Read the model definition and answer for the solid it produces. Units are mm, in the model's axes. Face numbers are marked on the shaded views. Give positions to 0.01 mm unless a question says otherwise; leave off trailing zeros. Order: outer loops, then holes, each group sorted by start corner. A loop starts at its lowest first (then second) coordinate and runs counter-clockwise, first axis right, second up. Notation, with made-up numbers: (50.5, -38) - (95.5, -38) arc R12 ccw to (95.5, -28) - close; hole circle Ø8 at (67.25, 71). An arc over 180 degrees is marked (long way). Return JSON: item names as keys, results as strings.
```python
from build123d import *

# Parameters (mm, degrees)
SHELL3_T           = 10
SKETCH5_R          = 8.5
CUT_EXTRUDE1_DEPTH = 10
CHAMFER2_SIZE      = 5


with BuildPart() as part:
    # Sketch4 → Loft3 section 0
    with BuildSketch(Plane(origin=(120, 0, 0), x_dir=(0, 0, -1), z_dir=(1, 0, 0))):
        with BuildLine():
            Line((13.75, 7.5), (-13.75, 7.5))
            Line((-13.75, 7.5), (-13.75, 32.5))
            Line((-13.75, 32.5), (13.75, 32.5))
            Line((13.75, 32.5), (13.75, 7.5))
        make_face()
    # Sketch1 → Loft3 section 1
    with BuildSketch(Plane(origin=(0, 0, 0), x_dir=(0, 0, -1), z_dir=(1, 0, 0))):
        with BuildLine():
            Line((-13.625, -12.5), (13.625, -12.5))
            Line((13.625, -12.5), (13.625, 12.5))
            Line((13.625, 12.5), (-13.625, 12.5))
            Line((-13.625, 12.5), (-13.625, -12.5))
        make_face()
    loft()

    # Shell3
    shell3_openings = [part.faces().sort_by_distance(p)[0] for p in [
        (60.091324201, 22.5152207, 0),
        (120, 20, 0),
    ]]
    offset(amount=SHELL3_T, openings=shell3_openings, kind=Kind.INTERSECTION)

    # Sketch5 → Cut-Extrude1 (cut)
    with BuildSketch(Plane(origin=(2.027027027, -12.162162162, 0), x_dir=(0.9863939238321439, 0.1643989873053572, 0), z_dir=(-0.1643989873053572, 0.9863939238321439, 0))):
        with Locations(Location((8.494520618, 0, 0), (0, 0, 180))):
            Circle(SKETCH5_R)
    extrude(amount=-CUT_EXTRUDE1_DEPTH, mode=Mode.SUBTRACT)

    # Chamfer2
    # the kernel refuses this chamfer: 5 mm, written as the material it takes off along each edge
    with BuildSketch(Plane(origin=(10.40597055, -10.765671575, 0), x_dir=(-0.9863939238321437, -0.1643989873053573, 0), z_dir=(0, 0, -1))) as chamfer2_piece_1_section:
        Polygon((8.5 + CHAMFER2_SIZE, 0), (8.5, -CHAMFER2_SIZE), (8.5, 0), align=None)
    chamfer2_piece_1 = revolve(axis=Axis((10.40597055, -10.765671575, 0), (-0.1643989873053572, 0.9863939238321439, 0)), mode=Mode.PRIVATE)
    chamfer2_piece_1 = split(chamfer2_piece_1, bisect_by=Plane(origin=(0, -11.368477015, 0), z_dir=(1, 0, 0)), keep=Keep.TOP, mode=Mode.PRIVATE)
    add(chamfer2_piece_1, mode=Mode.SUBTRACT)


solid = part.part
```
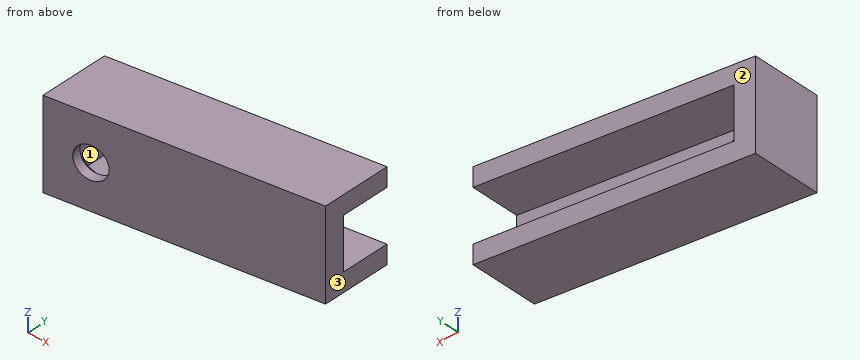
Q1. A cutting plane is placed at A-A (z = 20.5). Write down the section's boundary in (x, y).
Values:
{"outline": "(-10, -24.3) - (120, -2.64) - (120, 32.5) - (-10, 10.83) - close"}
Q2. Consider L1, parallel to Z at x = 108, y = 6; L2, parallel to Z at x = 105.5, y = 5; L3, parallel to Z at x = 21, y = 0. Determine where each line is inside the solid, lowest interval first.
Values:
{"L1": "z = -23.74 to -13.74, 13.74 to 23.74", "L2": "z = -23.73 to 23.73", "L3": "z = -23.65 to -13.65, 13.65 to 23.65"}
Q3. Given pin 1 (1.5 mm diameter, centred on x = 81, z = -1.5, fed in from -Y); pin 2 (8 mm diameter, centred on x = 44, z = 5, fed in from -Y); pin 3 (12 mm diameter, centred on x = 33.5, y = 1.5, fed in from -Z), each flat-ended and moving along its own axis, determine where each tip first touches the part or whether it passes through.
Values:
{"pin 1": "stops at y = -9.26", "pin 2": "stops at y = -15.97", "pin 3": "stops at z = -23.67"}
Q4. Determine the mould class of the marked faces 1, 2 and 3 for opening direction X: released by +X, released by -X, zero draft, split by the parting line, or undercut.
Values:
{"face 1": "undercut", "face 2": "released by -X", "face 3": "released by +X"}
